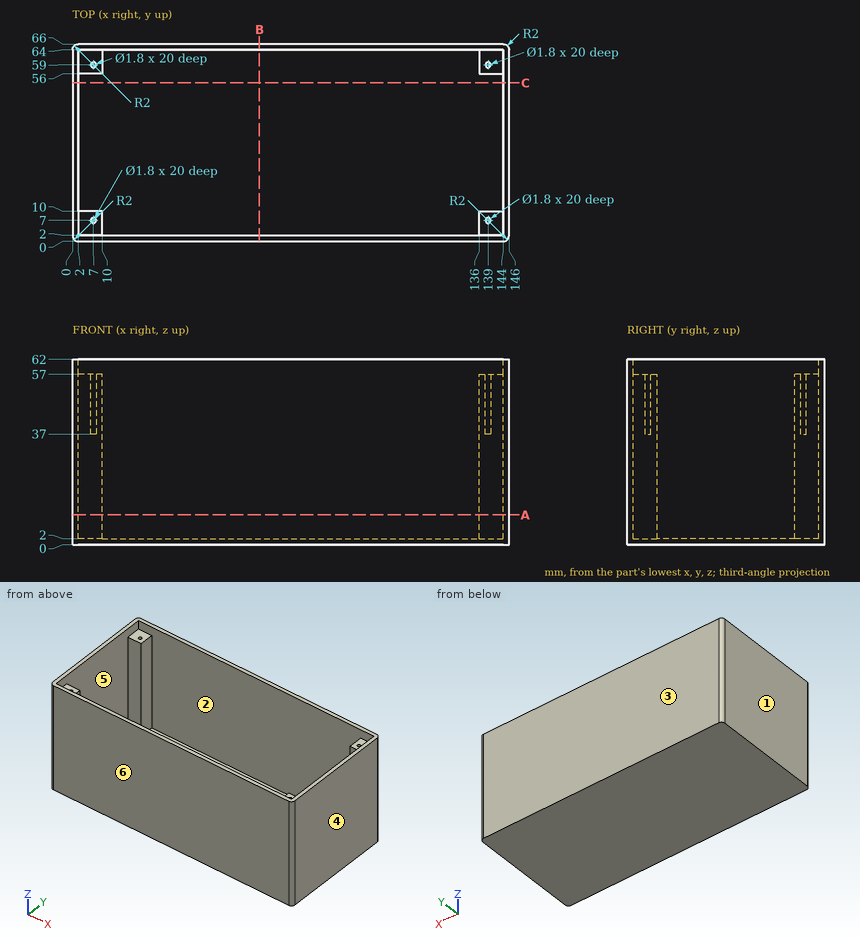
Print and shaded views of the part. All mm, measured from the part's lowest x, y and z. A direction names the side the tool comes from. Coordinates: 2 decimals unless noted, no trailing zeros. Loops run counter-clockwise (first coordinate to the right, second up) from the corner with the lowest first, then second, coordinate; pieces in that order, holes last. Notation, with made-up numbers: (86.25, 37.25) -> (123.25, 37.25) arc R7 cw to (123.25, 49.25) -> close; hole circle Ø7 at (37, 53). An arc over 180 degrees is marked (long way). Use a Markdown table: item, result. Add a question column.
Item 1: Probe probe 1 along X at (y, z) = (59, 41); probe 2 along Y at (x, z) = (139, 46.75); probe 3 along Y at (x, z) = (63.5, 22). List the from-to ranges inside material, lowest first.
Item 2: Pull direction Y, two halves, no side cores. Call the marked faces 3, 4, 5 and 6: +Y half, -Y half, draft (parallel to the pull), parting line (faces both ways), or undercut.
Item 3: Band-saw the part on B-B on x = 62.5. Write the cut outline in (y, z), plus the area to 3 significant figures.
Item 4: Which spindle directions (+Z, -Z, +X, -X, +Y, -Y) get a long thin tool onto all of the face, cutting with end or side? Do the marked faces 1 and 2. Say none if no direction does.
Item 5: Band-saw the part on C-C on y = 53. Write the cut outline in (x, z), plus the area to 3 significant figures.
Item 6: Band-saw the part on A-A on z = 10. Write the cut outline in (x, y), plus the area to 3 significant figures.
Item 7: Flat gauge pin, fed straight in: P1, Ø1.4, axis at x = 7, y = 7.5, coming from the +Z side. Where does the tip first touch, or does it go through?
Geometry says:
| question | item | result |
|---|---|---|
| 1 | probe 1 | 0 to 6.1, 7.9 to 10, 136 to 138.1, 139.9 to 146 |
| 1 | probe 2 | 0 to 6.1, 7.9 to 10, 56 to 58.1, 59.9 to 66 |
| 1 | probe 3 | 0 to 2, 64 to 66 |
| 2 | face 3 | +Y half |
| 2 | face 4 | draft |
| 2 | face 5 | undercut |
| 2 | face 6 | -Y half |
| 3 | outline | (0, 0) -> (66, 0) -> (66, 62) -> (64, 62) -> (64, 2) -> (2, 2) -> (2, 62) -> (0, 62) -> close |
| 3 | area | 372 mm² |
| 4 | face 1 | +Z, -Z, -X, +Y, -Y |
| 4 | face 2 | +Z |
| 5 | outline | (0, 0) -> (146, 0) -> (146, 62) -> (144, 62) -> (144, 2) -> (2, 2) -> (2, 62) -> (0, 62) -> close |
| 5 | area | 532 mm² |
| 6 | outline | (0, 2) arc R2 ccw to (2, 0) -> (144, 0) arc R2 ccw to (146, 2) -> (146, 64) arc R2 ccw to (144, 66) -> (2, 66) arc R2 ccw to (0, 64) -> close; hole (2, 10) -> (10, 10) -> (10, 2) -> (136, 2) -> (136, 10) -> (144, 10) -> (144, 56) -> (136, 56) -> (136, 64) -> (10, 64) -> (10, 56) -> (2, 56) -> close |
| 6 | area | 1,080 mm² |
| 7 | P1 | z = 57 |
